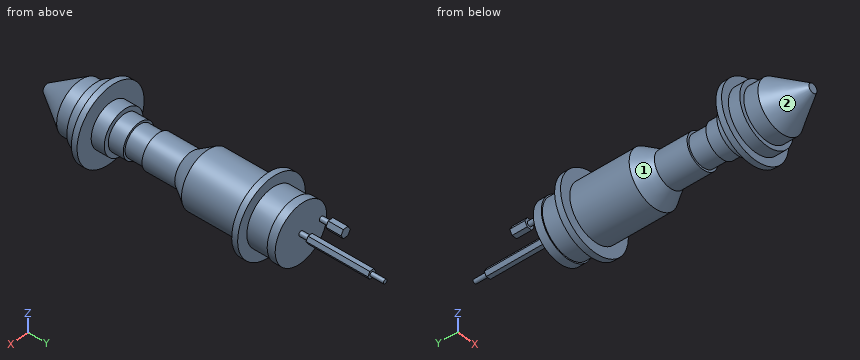
from build123d import *

# Parameters (mm, degrees)
SKETCH_2_R      = 4
EXTRUDE_1_DEPTH = 15
EXTRUDE_2_DEPTH = 102
SKETCH_4_R      = 3.42
EXTRUDE_3_DEPTH = 22
EXTRUDE_4_DEPTH = 25


with BuildPart() as part:
    # 草图1 → 旋转1 (revolve)
    with BuildSketch(Plane.XY, mode=Mode.PRIVATE) as revolve_1_sk:
        Polygon((0, 0), (7.5, 0), (42.09, 53.35), (42.09, 76.73), (49.525, 76.73), (49.525, 95.5), (62.215, 95.5), (62.215, 104.91), (36.02, 104.91), (36.02, 126.55), (28.645, 126.55), (28.645, 151.31), (25.25, 151.31), (25.25, 182.28), (28.645, 182.28), (28.645, 236.27), (45.765, 262.67), (45.765, 360.73), (62.835, 360.73), (62.835, 370.54), (45.765, 370.54), (45.765, 405.93), (47.82, 405.93), (47.82, 419.14), (0, 419.14), align=None)
    revolve(revolve_1_sk.sketch.rotate(Axis((0, 0, 0), (0, 1, 0)), 90), axis=Axis((0, 0, 0), (0, 1, 0)))

    # 草图2 → 凸台-拉伸1 (add)
    with BuildSketch(Plane(origin=(0, 419.14, 0), x_dir=(1, 0, 0), z_dir=(0, 1, 0))):
        with Locations(Location((0, 0, 0), (0, 0, 270))):
            Circle(SKETCH_2_R)
        with Locations(Location((-38, 0, 0), (0, 0, 270))):
            Circle(SKETCH_2_R)
    extrude(amount=EXTRUDE_1_DEPTH)

    # 草图3 → 凸台-拉伸2 (add)
    with BuildSketch(Plane(origin=(0, 434.14, 0), x_dir=(1, 0, 0), z_dir=(0, 1, 0))):
        Polygon((3.674834463, -6.365), (7.349668927, 0), (3.674834463, 6.365), (-3.674834463, 6.365), (-7.349668927, 0), (-3.674834463, -6.365), align=None)
    extrude(amount=EXTRUDE_2_DEPTH)

    # 草图4 → 凸台-拉伸3 (add)
    with BuildSketch(Plane(origin=(0, 536.14, 0), x_dir=(1, 0, 0), z_dir=(0, 1, 0))):
        with Locations(Location((0, 0, 0), (0, 0, 270))):
            Circle(SKETCH_4_R)
    extrude(amount=EXTRUDE_3_DEPTH)

    # 草图5 → 凸台-拉伸4 (add)
    with BuildSketch(Plane(origin=(0, 434.14, 0), x_dir=(1, 0, 0), z_dir=(0, 1, 0))):
        Polygon((-29.449442513, 0), (-33.724721257, 7.405), (-42.275278743, 7.405), (-46.550557487, 0), (-42.275278743, -7.405), (-33.724721257, -7.405), align=None)
    extrude(amount=EXTRUDE_4_DEPTH)


solid = part.part
Could you check a few things on this model? Use its own coordinates, in mm. Face numbers are marked on the shaded views. Coordinates: 2 decimals unless noted, no trailing zeros. Order: outer loops, then holes, each group sorted by start corner. A loop starts at its lowest first (then second) coordinate and runs counter-clockwise, first axis right, second up. Notation, with made-up numbers: (-31, 50.25) - (-14, 50.25) arc R20 cw to (-14, 76.25) - close; hole circle Ø11 at (72.5, 56.5). An arc over 180 degrees is marked (long way). Answer in a Markdown table with one row per item. Add a question column.
(1) If we mould it in two halves opening along Y, with no side actions, what happens to the marked faces 1 and 2? For each: released by +Y, released by -Y, zero draft, split by the parting line, or undercut.
(2) I need wall thicknesses on L1, parallel to Y at x = -52.5, z = -16; L2, parallel to Y at x = -42.5, z = 22; L3, parallel to Y at x = -13, z = -17.5. Which ranges of each line are inside material? Lowest first, please.
(3) If we section it at A-A, the plane y = 200.5: Please give me the cut outline in (x, z) (3 decimals).
(4) Will these pins go through, and if not, where does the flat tip stop? pin 1 (2 mm diameter, centred on y = 141, z = 1.5, fed in from +X); pin 2 (12 mm diameter, centred on x = -40, z = -3, fed in from -Y); pin 3 (1 mm diameter, centred on y = 230, z = 25, fed in from +X).
Results are:
| question | item | result |
|---|---|---|
| 1 | face 1 | undercut |
| 1 | face 2 | released by -Y |
| 2 | L1 | y = 95.5 to 104.91, 360.73 to 370.54 |
| 2 | L2 | y = 76.73 to 104.91, 360.73 to 370.54 |
| 2 | L3 | y = 22.06 to 419.14 |
| 3 | outline | circle Ø57.29 at (0, 0) |
| 4 | pin 1 | stops at x = 28.64 |
| 4 | pin 2 | stops at y = 41.05 |
| 4 | pin 3 | stops at x = 14.84 |
